Read the model definition and answer for the solid it produces. Units are mm, in the model's axes. A direction names the side the tool comes from. Coordinates: 2 decimals unless noted, no trailing zeros. Loops run counter-clockwise (first coordinate to the right, second up) from the corner with the lowest first, then second, coordinate; pieces in that order, holes last.
from build123d import *

# Parameters (mm, degrees)
SKETCH_1_W          = 600
SKETCH_1_H          = 2200
EXTRUDE_1_DEPTH     = 485
SKETCH_2_W          = 230
SKETCH_2_H          = 1360
CUT_EXTRUDE_1_DEPTH = 135
SKETCH_3_W          = 230
SKETCH_3_H          = 390
CUT_EXTRUDE_2_DEPTH = 445
SKETCH_4_W          = 230
SKETCH_4_H          = 340
CUT_EXTRUDE_3_DEPTH = 445
SKETCH_5_W          = 580
SKETCH_5_H          = 290
EXTRUDE_2_DEPTH     = 20
FILLET_1_R          = 50
SKETCH_6_W          = 230
SKETCH_6_H          = 610
CUT_EXTRUDE_4_DEPTH = 20
SKETCH_7_W          = 240
SKETCH_7_H          = 620
EXTRUDE_3_DEPTH     = 20
FILLET_2_R          = 50
FILLET_3_R          = 50


with BuildPart() as part:
    # 스케치1 → 보스-돌출1 (new body)
    with BuildSketch(Plane.XY):
        Rectangle(SKETCH_1_W, SKETCH_1_H)
    extrude(amount=-EXTRUDE_1_DEPTH)

    # 스케치2 → 컷-돌출1 (cut)
    with BuildSketch(Plane(origin=(300, 0, 0), x_dir=(0, 0, -1), z_dir=(1, 0, 0))):
        with Locations((370, 420)):
            Rectangle(SKETCH_2_W, SKETCH_2_H)
    extrude(amount=-CUT_EXTRUDE_1_DEPTH, mode=Mode.SUBTRACT)

    # 스케치3 → 컷-돌출2 (cut)
    with BuildSketch(Plane(origin=(165, 0, 0), x_dir=(0, 0, -1), z_dir=(1, 0, 0))):
        with Locations((370, -65)):
            Rectangle(SKETCH_3_W, SKETCH_3_H)
    extrude(amount=-CUT_EXTRUDE_2_DEPTH, mode=Mode.SUBTRACT)

    # 스케치4 → 컷-돌출3 (cut)
    with BuildSketch(Plane(origin=(165, 0, 0), x_dir=(0, 0, -1), z_dir=(1, 0, 0))):
        with Locations((370, 320)):
            Rectangle(SKETCH_4_W, SKETCH_4_H)
    extrude(amount=-CUT_EXTRUDE_3_DEPTH, mode=Mode.SUBTRACT)

    # 스케치5 → 보스-돌출2 (add)
    with BuildSketch(Plane(origin=(0, -260, 0), x_dir=(1, 0, 0), z_dir=(0, 1, 0))):
        with Locations((10, 400)):
            Rectangle(SKETCH_5_W, SKETCH_5_H)
    extrude(amount=EXTRUDE_2_DEPTH)

    # 필렛1
    fillet_1_edges = [part.edges().sort_by_distance(p)[0] for p in [
        (300, -250, -545),
    ]]
    fillet(fillet_1_edges, radius=FILLET_1_R)

    # 스케치6 → 컷-돌출4 (cut)
    with BuildSketch(Plane(origin=(165, 0, 0), x_dir=(0, 0, -1), z_dir=(1, 0, 0))):
        with Locations((370, 795)):
            Rectangle(SKETCH_6_W, SKETCH_6_H)
    extrude(amount=-CUT_EXTRUDE_4_DEPTH, mode=Mode.SUBTRACT)

    # 스케치7 → 보스-돌출3 (add)
    with BuildSketch(Plane(origin=(145, 0, 0), x_dir=(0, 0, -1), z_dir=(1, 0, 0))):
        with Locations((375, 790)):
            Rectangle(SKETCH_7_W, SKETCH_7_H)
    extrude(amount=EXTRUDE_3_DEPTH)

    # 필렛2
    fillet_2_edges = [part.edges().sort_by_distance(p)[0] for p in [
        (-280, -250, -545),
    ]]
    fillet(fillet_2_edges, radius=FILLET_2_R)

    # 필렛3
    fillet_3_edges = [part.edges().sort_by_distance(p)[0] for p in [
        (165, 140, -485),
    ]]
    fillet(fillet_3_edges, radius=FILLET_3_R)


solid = part.part
Q1. Which of the six approach directions +Z, -Z, +X, -X, +Y, -Y give full straight-line access (tool end or side, diameter ignored) to faces 1 (the face through (-280, -52, -368)), 2 (the face through (-65, 490, -368)), 3 (the face through (-4, 15, 0))?
Findings below:
face 1: -Z, +X
face 2: -Z
face 3: +Z, +X, -X, +Y, -Y
Q2. Determine the mould class of faces 4 (the face through (165, 794, -373)), 5 (the face through (-54, 150, -368)), 6 (the face through (6, -260, -515)) for opening direction Y: +Y half, -Y half, draft (parallel to the pull), parting line (faces both ways), or undercut.
Findings below:
face 4: draft
face 5: undercut
face 6: -Y half
Q3. A cutting plane is placed at A-A (z = -346). Give the vertices of the cut face in (x, y).
Findings below:
outline: (-300, -1100) - (300, -1100) - (300, -240) - (-280, -240) - (-280, 130) - (165, 130) - (165, 150) - (-280, 150) - (-280, 490) - (145, 490) - (145, 480) - (165, 480) - (165, 1100) - (-300, 1100) - close
Q4. Flat-ended cylindrical pins translate along their axes: pin 1 Ø2 at (x, z) = (176, -480.5) entering from +Y; pin 2 Ø5 at (y, z) = (-255, -489) entering from -X; pin 3 Ø16 at (y, z) = (140.5, -351) entering from +X. Find the tip coordinate at first contact, or state that the pin passes through.
Findings below:
pin 1: stops at y = -240
pin 2: stops at x = -280
pin 3: stops at x = 165
Q5. Straight lines are drawn through the part: probe 1 along Y at (x, z) = (140, -262); probe 2 along Z at (x, y) = (122, 0.5); probe 3 along Z at (x, y) = (12.5, -830.5). For each, find the intervals that lie inside material, in ascending order.
Findings below:
probe 1: y = -1100 to -240, 130 to 150, 490 to 1100
probe 2: z = -255 to 0
probe 3: z = -485 to 0
Q6. A cutting plane is placed at C-C (y = -31). Give the vertices of the cut face in (x, z), then the cut area to 3 significant figures.
Findings below:
outline: (-300, -485) - (-280, -485) - (-280, -255) - (300, -255) - (300, 0) - (-300, 0) - close
area: 158,000 mm2
Q7. A cutting plane is placed at D-D (x = -100). Give the vertices of the cut face in (y, z), then the cut area to 3 significant figures.
Findings below:
outline: (-1100, -485) - (-260, -485) - (-260, -545) - (-240, -545) - (-240, -255) - (130, -255) - (130, -485) - (150, -485) - (150, -255) - (490, -255) - (490, -485) - (1100, -485) - (1100, 0) - (-1100, 0) - close
area: 905,000 mm2
Q8. A cutting plane is placed at B-B (x = 220.5). Give the vertices of the cut face in (y, z).
Findings below:
outline: (-1100, -485) - (-260, -485) - (-260, -545) - (-240, -545) - (-240, -255) - (1100, -255) - (1100, 0) - (-1100, 0) - close
